The listing builds one solid part. Answer for the finished solid, in the listing's coordinates (mm). Face numbers are marked on the shaded views. A direction names the side the tool comes from. Round coordinates to 2 decimals unless told otherwise and drop trailing zeros. Loops run counter-clockwise (first coordinate to the right, second up) from the corner with the lowest first, then second, coordinate; pieces in that order, holes last. Notation, with made-up numbers: M 79,5 L 98,5 A19 cw 98,37 Z; hole C -39,-38 d8. An arc over 180 degrees is marked long. Put each result on its own line as item: value. Start each with the question number.
(1) Section D-D, the plane x = 4.25 is taken. Determine the outline of the cut face in (y, z).
(2) Section C-C, the plane x = -3 is taken. Determine the outline of the cut face in (y, z).
(3) Straight lines are drawn through the part: line 1 (X direction, y = 4.05, z = 3.9); line 2 (X direction, y = 2.15, z = -5.5); line 3 (Z direction, x = -8, y = 4.05). For each, find the intervals that lie inside material, in ascending order.
(4) Flat-ended cylindrical pins translate along their axes: P1, Ø1.1, axis at y = 2, z = -5.5, coming from the +X side; P2, Ø1.5, axis at x = 6, y = 2.5, coming from the +Z side; P3, Ø3, axis at x = 7, y = 3.5, coming from the -Z side. Find the tip coordinate at first contact, or state that the pin passes through.
(5) Section B-B, the plane z = -4.5 is taken. Determine the outline of the cut face in (x, y), then the cut area to 3 significant figures.
(6) Which of the six approach directions +Z, -Z, +X, -X, +Y, -Y give full straight-line access (tool end or side, diameter ignored) to the marked faces 1, 2 and 3?
(7) Section A-A, the plane y = 3.2 is taken. Determine the outline of the cut face in (x, z), then the cut area to 3 significant figures.
(8) Determine the mould class of the marked faces 4, 5 and 6 for opening direction Z: released by +Z, released by -Z, zero draft, split by the parting line, or undercut.
```python
from build123d import *

# Parameters (mm, degrees)
EXTRUDE_1_DEPTH              = 1
EXTRUDE_3_DEPTH              = 4.2
EXTRUDE_3_DEPTH_BACK         = 1
SKETCH_5_R                   = 2.0000000000000004
SKETCH_5_R_2                 = 1.9999999999999996
SKETCH_7_R                   = 1.0299999999999991
EXTRUDE_4_DEPTH              = 4
HOLE_WIZARD_M2_1_D           = 1.6
HOLE_WIZARD_M2_1_DEPTH       = 4
HOLE_WIZARD_M2_1_CSINK_D     = 2.05
HOLE_WIZARD_M2_1_CSINK_ANGLE = 90
HOLE_WIZARD_M2_1_TIP         = 0.48068849522204826
CUT_EXTRUDE_1_DEPTH          = 14.435955492632447
CHAMFER_1_SIZE               = 0.2
CHAMFER_2_SIZE               = 0.2


with BuildPart() as part:
    # 草图1 → 凸台-拉伸1 (new body)
    with BuildSketch(Plane(origin=(0, 0, 0), x_dir=(1, 0, 0), z_dir=(0, 1, 0))):
        Polygon((-10.000000000000002, 5.4), (9.999999999999998, 5.4), (9.999999999999998, -5.4), (-10, -5.4), align=None)
    extrude(amount=EXTRUDE_1_DEPTH)

    # 草图5 → 凸台-拉伸3 (add, two sides: drawn at the far end of the back side and taken through both)
    with BuildSketch(Plane(origin=(0, 1, 0), x_dir=(1, 0, 0), z_dir=(0, 1, 0)).offset(-EXTRUDE_3_DEPTH_BACK)):
        with Locations(Location((-8.000000000000002, -3.900000000000001, 0), (0, 0, 270))):
            Circle(SKETCH_5_R)
        with Locations(Location((7.999999999999998, -3.900000000000001, 0), (0, 0, 270))):
            Circle(SKETCH_5_R_2)
    extrude(amount=EXTRUDE_3_DEPTH + EXTRUDE_3_DEPTH_BACK)

    # 草图7 → 凸台-拉伸4 (add)
    with BuildSketch(Plane(origin=(0, 1, 0), x_dir=(1, 0, 0), z_dir=(0, 1, 0))):
        with BuildLine():
            Line((-1.9700000000000024, 5.4), (-4.030000000000003, 5.4))
            Line((-4.030000000000002, 5.4), (-4.030000000000001, 1.3999999999999986))
            ThreePointArc((-4.030000000000002, 1.3999999999999988), (-3.0000000000000018, 2.429999999999999), (-1.9700000000000017, 1.3999999999999986))
            Line((-1.9700000000000017, 1.3999999999999986), (-1.9700000000000022, 5.4))
        make_face()
        with BuildLine():
            ThreePointArc((-1.9700000000000017, 1.3999999999999986), (-3.0000000000000018, 2.429999999999999), (-4.030000000000002, 1.3999999999999988))
            Line((-4.030000000000001, 1.3999999999999986), (-1.9700000000000015, 1.3999999999999986))
        make_face()
        with BuildLine():
            Line((-1.9700000000000015, 1.3999999999999986), (-4.030000000000001, 1.3999999999999986))
            ThreePointArc((-4.030000000000002, 1.3999999999999988), (-3.0000000000000018, 0.36999999999999855), (-1.9700000000000017, 1.3999999999999984))
        make_face()
        with BuildLine():
            Line((4.029999999999997, 5.4), (1.9699999999999989, 5.4))
            Line((1.9699999999999989, 5.4), (1.9700000000000004, 1.4000000000000021))
            ThreePointArc((1.9699999999999973, 1.400000000000002), (2.9999999999999982, 2.4300000000000024), (4.029999999999999, 1.4000000000000017))
            Line((4.029999999999997, 1.4000000000000021), (4.029999999999997, 5.4))
        make_face()
        with BuildLine():
            ThreePointArc((4.029999999999999, 1.4000000000000017), (2.9999999999999982, 2.4300000000000024), (1.9699999999999973, 1.400000000000002))
            Line((1.9700000000000004, 1.4000000000000015), (4.029999999999997, 1.400000000000002))
        make_face()
        with BuildLine():
            Line((4.029999999999997, 1.400000000000002), (1.9700000000000004, 1.4000000000000015))
            ThreePointArc((1.9699999999999973, 1.400000000000002), (2.9999999999999982, 0.3700000000000008), (4.029999999999999, 1.4000000000000015))
        make_face()
        with BuildLine():
            ThreePointArc((-1.9700000000000022, 6.8999999999999995), (-3.0000000000000013, 5.87), (-4.03, 6.8999999999999995))
            Line((-4.030000000000002, 6.8999999999999995), (-4.030000000000002, 5.4))
            Line((-4.030000000000003, 5.4), (-1.9700000000000024, 5.4))
            Line((-1.9700000000000022, 5.4), (-1.9700000000000024, 6.8999999999999995))
        make_face()
        with Locations((-3.0000000000000013, 6.8999999999999995)):
            Circle(SKETCH_7_R)
        with BuildLine():
            Line((1.9699999999999982, 6.899999999999999), (1.9699999999999989, 5.4))
            Line((1.9699999999999989, 5.4), (4.029999999999997, 5.4))
            Line((4.029999999999997, 5.4), (4.029999999999997, 6.8999999999999995))
            ThreePointArc((4.029999999999998, 6.8999999999999995), (2.9999999999999982, 5.87), (1.969999999999999, 6.8999999999999995))
        make_face()
        with Locations((2.9999999999999982, 6.8999999999999995)):
            Circle(SKETCH_7_R)
    extrude(amount=EXTRUDE_4_DEPTH)

    # M2 螺纹孔1
    with Locations(Plane(origin=(0, 5.200000000000001, 0), x_dir=(1, 0, 0), z_dir=(0, 1, 0))):
        with Locations((-8, -3.9), (8, -3.9)):
            CounterSinkHole(HOLE_WIZARD_M2_1_D / 2, HOLE_WIZARD_M2_1_CSINK_D / 2, depth=HOLE_WIZARD_M2_1_DEPTH, counter_sink_angle=HOLE_WIZARD_M2_1_CSINK_ANGLE)
            with Locations((0, 0, -(HOLE_WIZARD_M2_1_DEPTH + HOLE_WIZARD_M2_1_TIP / 2))):  # 118° drill point
                Cone(0, HOLE_WIZARD_M2_1_D / 2, HOLE_WIZARD_M2_1_TIP, mode=Mode.SUBTRACT)

    # 草图10 → 切除-拉伸1 (cut, through all)
    with BuildSketch(Plane(origin=(0, 1, 0), x_dir=(1, 0, 0), z_dir=(0, 1, 0))):
        with BuildLine():
            Line((-10.000000000000002, -5.3999999999999995), (-9.322875655532316, -5.3999999999999995))
            ThreePointArc((-9.322875655532314, -5.399999999999986), (-9.822875655532302, -4.722875655532286), (-10.000000000000002, -3.9000000000000004))
            Line((-10.000000000000002, -3.900000000000002), (-10.000000000000002, -5.3999999999999995))
        make_face()
        with BuildLine():
            Line((9.322875655532266, -5.3999999999999995), (9.999999999999998, -5.3999999999999995))
            Line((9.999999999999998, -5.3999999999999995), (9.999999999999998, -3.900000000000001))
            ThreePointArc((9.999999999999998, -3.9000000000000012), (9.822875655532286, -4.7228756555323095), (9.322875655532272, -5.400000000000019))
        make_face()
    extrude(amount=-CUT_EXTRUDE_1_DEPTH, mode=Mode.SUBTRACT)

    # 倒角1
    # the kernel refuses this chamfer: 0.2 mm, written as the material it takes off along each edge
    with BuildSketch(Plane(origin=(-10, 1, 4.414336597593362), x_dir=(-0.02749587661058736, -0.9996219169112966, 0), z_dir=(-1.6e-16, 0, -1))) as chamfer_1_piece_1_section:
        Polygon((CHAMFER_1_SIZE * 0.999621916911, -CHAMFER_1_SIZE * 0.0274958766106), (-CHAMFER_1_SIZE * 0.0274958766106, -CHAMFER_1_SIZE * 0.999621916911), (0, 0), align=None)
    chamfer_1_piece_1 = extrude(amount=10.328673195186546, mode=Mode.PRIVATE)
    chamfer_1_piece_1 = chamfer_1_piece_1 - Plane(origin=(-8.000000000000002, 0.9330678370118787, 3.900000000000001), x_dir=(-1.8e-16, 0, 1), z_dir=(0, -1, 0)) * Cylinder(2.0000000000000004, 22, mode=Mode.PRIVATE)
    add(chamfer_1_piece_1, mode=Mode.SUBTRACT)
    with BuildSketch(Plane(origin=(9.999999999999998, 1, -5.9143365975931825), x_dir=(0.02749587661058736, -0.9996219169112966, 0), z_dir=(0, 0, 1))) as chamfer_1_piece_2_section:
        Polygon((CHAMFER_1_SIZE * 0.999621916911, -CHAMFER_1_SIZE * 0.0274958766106), (-CHAMFER_1_SIZE * 0.0274958766106, -CHAMFER_1_SIZE * 0.999621916911), (0, 0), align=None)
    chamfer_1_piece_2 = extrude(amount=10.328673195185887, mode=Mode.PRIVATE)
    chamfer_1_piece_2 = chamfer_1_piece_2 - Plane(origin=(7.999999999999998, 0.9330678369662879, 3.900000000000001), x_dir=(-1.8e-16, 0, 1), z_dir=(0, -1, 0)) * Cylinder(1.9999999999999996, 22, mode=Mode.PRIVATE)
    add(chamfer_1_piece_2, mode=Mode.SUBTRACT)
    with BuildSketch(Plane(origin=(-10.000000000000002, -0.5143365975931808, -5.4), x_dir=(0.9996219169112966, 0, -0.02749587661058742), z_dir=(0, 1, 0))) as chamfer_1_piece_3:
        Polygon((CHAMFER_1_SIZE * 0.999621916911, -CHAMFER_1_SIZE * 0.0274958766106), (-CHAMFER_1_SIZE * 0.0274958766106, -CHAMFER_1_SIZE * 0.999621916911), (0, 0), align=None)
    extrude(amount=2.0286731951863617, mode=Mode.SUBTRACT)
    with BuildSketch(Plane(origin=(9.999999999999998, -0.5143365975931831, -5.4), x_dir=(-0.9996219169112966, 0, -0.02749587661058742), z_dir=(0, 1, 0))) as chamfer_1_piece_4:
        Polygon((CHAMFER_1_SIZE * 0.999621916911, CHAMFER_1_SIZE * 0.0274958766106), (-CHAMFER_1_SIZE * 0.0274958766106, CHAMFER_1_SIZE * 0.999621916911), (0, 0), align=None)
    extrude(amount=2.028673195186366, mode=Mode.SUBTRACT)

    # 倒角2
    chamfer_2_edges = [part.edges().sort_by_distance(p)[0] for p in [
        (-1.970000000000002, 5, -4.149999999999999),
        (-4.030000000000001, 5, -4.149999999999999),
        (-3.000000000000002, 5, -0.3699999999999988),
        (-3.0000000000000013, 5, -7.929999999999999),
        (4.029999999999998, 5, -4.15),
        (1.9699999999999986, 5, -4.15),
        (2.999999999999998, 5, -0.3700000000000008),
        (2.9999999999999982, 5, -7.929999999999999),
    ]]
    chamfer(chamfer_2_edges, length=CHAMFER_2_SIZE)


solid = part.part
```
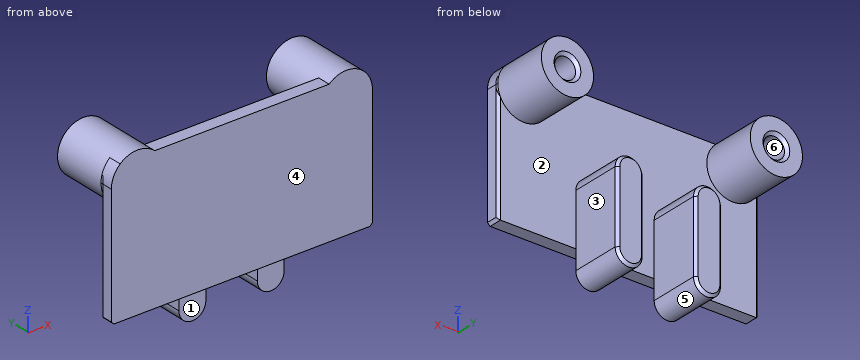
Recorded:
1. outline: M 0,-5.4 L 1,-5.4 L 1,5.4 L 0,5.4 Z
2. outline: M 0,-5.4 L 1,-5.4 L 1,-7.93 L 4.8,-7.93 L 5,-7.73 L 5,-0.57 L 4.8,-0.37 L 1,-0.37 L 1,5.4 L 0,5.4 Z
3. line 1: x = -10 to -8.8, -7.2 to -6, 6 to 7.2, 8.8 to 10
3. line 2: x = -4.03 to -1.97, 1.97 to 4.03
3. line 3: z = 1.9 to 3.1, 4.7 to 5.9
4. P1: stops at x = 4.03
4. P2: stops at z = 5.46
4. P3: stops at z = 1.9
5. outline: M -10,0 L 10,0 L 10,0.8 L 9.8,1 L 4.03,1 L 4.03,4.8 L 3.83,5 L 2.17,5 L 1.97,4.8 L 1.97,1 L -1.97,1 L -1.97,4.8 L -2.17,5 L -3.83,5 L -4.03,4.8 L -4.03,1 L -9.8,1 L -10,0.8 Z
5. area: 36.4 mm²
6. face 1: -Z, +X, -X, -Y
6. face 2: +Y
6. face 3: +Z, -Z, +X, +Y
7. outline: C -8,3.9 d4; M -4.03,-6.9 A1.03 ccw -1.97,-6.9 L -1.97,-1.4 A1.03 ccw -4.03,-1.4 Z; M 1.97,-6.9 A1.03 ccw 4.03,-6.9 L 4.03,-1.4 A1.03 ccw 1.97,-1.4 Z; C 8,3.9 d4; hole C -8,3.9 d1.6; hole C 8,3.9 d1.6
7. area: 50.4 mm²
8. face 4: zero draft
8. face 5: released by -Z
8. face 6: undercut
